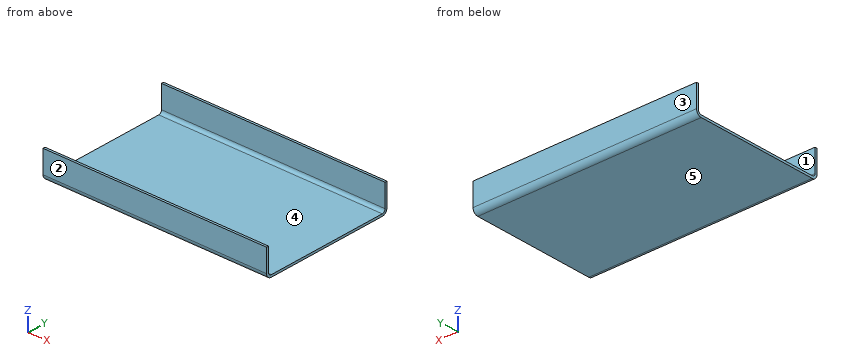
Autodesk Inventor part; units mm, degrees
ref_plane "YZ Plane" through (0, 0, 0) normal (1, 0, 0) x (0, 1, 0)
ref_plane "XZ Plane" through (0, 0, 0) normal (0, 1, 0) x (-1, 0, 0)
ref_plane "XY Plane" through (0, 0, 0) normal (0, 0, 1) x (1, 0, 0)
sketch "Sketch1" plane through (0, 0, 0) normal (0, 0, 1) x (1, 0, 0)
  line L0 (-100, -60) -> (100, -60)
  line L1 (100, -60) -> (100, 60)
  line L2 (100, 60) -> (-100, 60)
  line L3 (-100, 60) -> (-100, -60)
  line L4 (-100, -60) -> (100, 60) construction
  line L5 (100, -60) -> (-100, 60) construction
  point P0 (0, 0)
  dimension "d0" = 200
  dimension "d1" = 120
extrude "Plate1" add sketch "Sketch1" along normal blind 2
sketch "Sketch2" plane through (0, 0, 0) normal (0, 0, -1) x (-1, 0, 0)
  line L0 (-80, 40) -> (120, 40) construction
  line L1 (120, 40) -> (120, 20) construction
  line L2 (120, 20) -> (-80, 20) construction
  line L3 (-80, 20) -> (-80, 40) construction
  line L4 (-100, 60) -> (100, 60)
  line L5 (-100, -60) -> (-100, 60)
  point P0 (0, 0)
  point P1 (-48, 100)
  point P2 (-50, 98)
  dimension "d6" = 200
  dimension "d9" = 20
  dimension "d10" = 20
  dimension "d11" = 20
mark "Mark1"
sketch "Sketch3" plane through (100, 58, 0) normal (0, 1, 0) x (-1, 0, 0)
  line L0 (200, 0) -> (0, 0)
  line L1 (0, 0) -> (0, -25)
  line L2 (0, -25) -> (200, -25)
  line L3 (200, -25) -> (200, 0)
edge flange "Flange1" height 25 angle 90 thickness 2 bend radius 2.75 thickness toward (0, 1, 0) relief round relief width 2 relief depth 1 corner gap 2.75 corner form 0 edges at (0, 60, 0) (0, -60, 0) wall of the first edge with corners at (-100, 58, 0) (100, 58, 0) (100, 58, 25) (-100, 58, 25)
bend "Bend1"
corner "Corner1"
equation "\"d2\" = Thickness"
equation "\"d12\" = BendReliefWidth"
equation "\"d13\" = BendReliefDepth"
equation "\"d14\" = MinimumRemnant"
equation "\"d15\" = TransitionRadius"
equation "\"d18\" = BendRadius"
equation "\"d19\" = CornerReliefSize"
equation "\"d20\" = GapSize"
equation "\"d21\" = JacobiRadiusSize"
equation "\"BendReliefWidth\" = Thickness"
equation "\"BendReliefDepth\" = 0.5 * Thickness"
equation "\"CornerReliefSize\" = 4 * Thickness"
equation "\"MinimumRemnant\" = 2 * Thickness"
equation "\"TransitionRadius\" = BendRadius"
equation "\"JacobiRadiusSize\" = BendRadius"
equation "\"GapSize\" = Thickness"
properties part number "TRM 037 box 2" material "AISI 304"
Design review of the part built by this model. Coordinates are the model's own, in mm. Face numbers are marked on the shaded views. A direction names the side the tool comes from. Coordinates: 2 decimals unless noted, no trailing zeros. Order: outer loops, then holes, each group sorted by start corner. A loop starts at its lowest first (then second) coordinate and runs counter-clockwise, first axis right, second up. Notation, with made-up numbers: (51, 7) -> (83, 7) arc R8 ccw to (83, 20) -> close; hole circle Ø10 at (69.25, 16.25). An arc over 180 degrees is marked (long way). One line per item, written item: value.
1) Clearance check with flat-ended pins moving along their axes: P1, Ø4, axis at x = -65, y = -17.5, coming from the -Z side; P2, Ø1.5, axis at x = -36, y = -11, coming from the +Z side. State where each tip first meets the part, or that it passes through.
Output values:
P1: stops at z = 0
P2: stops at z = 2
2) Draft analysis for pull direction Y (two halves, no side actions). For the marked faces 1, 2 and 3, state which applies: +Y half, -Y half, draft (parallel to the pull), parting line (faces both ways), or undercut.
Output values:
face 1: undercut
face 2: -Y half
face 3: +Y half
3) Machinability: for the marked faces 4 and 5, which of the approach directions +Z, -Z, +X, -X, +Y, -Y give a long, thin tool a straight path to every point of the face, cutting with its end or side? Answer none if there is none.
Output values:
face 4: +Z, +X, -X
face 5: -Z, +X, -X, +Y, -Y
4) To check wall thickness, follow probe 1 along Y at (x, z) = (79, 12.5); probe 2 along Z at (x, y) = (33, 40.5); probe 3 along Y at (x, z) = (-59.5, 1). State the ranges of each line that lie inside material, in increasing order. Write a range as [from, to].
Output values:
probe 1: y = [-60, -58], [58, 60]
probe 2: z = [0, 2]
probe 3: y = [-58.17, 58.17]
5) We need section A-A, the plane z = 13.75. Give the boundary of the cut face in (x, y).
Output values:
outline: (-100, -60) -> (100, -60) -> (100, -58) -> (-100, -58) -> close; (-100, 58) -> (100, 58) -> (100, 60) -> (-100, 60) -> close
6) We need section C-C, the plane y = 13. Give the boundary of the cut face in (x, z).
Output values:
outline: (-100, 0) -> (100, 0) -> (100, 2) -> (-100, 2) -> close
7) We need section B-B, the plane x = -53. Give the boundary of the cut face in (y, z), then the cut area to 3 significant figures.
Output values:
outline: (-60, 4.75) arc R4.75 ccw to (-55.25, 0) -> (55.25, 0) arc R4.75 ccw to (60, 4.75) -> (60, 25) -> (58, 25) -> (58, 4.75) arc R2.75 cw to (55.25, 2) -> (-55.25, 2) arc R2.75 cw to (-58, 4.75) -> (-58, 25) -> (-60, 25) -> close
area: 326 mm2
